The model under review builds one solid part; all positions refer to its coordinate system, in mm. Coordinates: 2 decimals unless noted, no trailing zeros. Use one line per item in the form item = value.
```python
from build123d import *

# Parameters (mm, degrees)
F0_W     = 282
F0_H     = 90
F0_R     = 1.85
F0_R_2   = 4
F1_DEPTH = 3


with BuildPart() as f1:
    # F0 (on Top) → F1 (new body)
    with BuildSketch(Plane.XY):
        Rectangle(F0_W, F0_H)
        with Locations((-136, -40)):
            Circle(F0_R, mode=Mode.SUBTRACT)
        with Locations((-120, -40)):
            Circle(F0_R, mode=Mode.SUBTRACT)
        with Locations((-104, -40)):
            Circle(F0_R, mode=Mode.SUBTRACT)
        with Locations((-88, -40)):
            Circle(F0_R, mode=Mode.SUBTRACT)
        with Locations((-72, -40)):
            Circle(F0_R, mode=Mode.SUBTRACT)
        with Locations((-56, -40)):
            Circle(F0_R, mode=Mode.SUBTRACT)
        with Locations((-40, -40)):
            Circle(F0_R, mode=Mode.SUBTRACT)
        with Locations((-24, -40)):
            Circle(F0_R, mode=Mode.SUBTRACT)
        with Locations((-8, -40)):
            Circle(F0_R, mode=Mode.SUBTRACT)
        with Locations((-128, -8)):
            Circle(F0_R, mode=Mode.SUBTRACT)
        with Locations((-96, -8)):
            Circle(F0_R, mode=Mode.SUBTRACT)
        with Locations((-64, -8)):
            Circle(F0_R, mode=Mode.SUBTRACT)
        with Locations((-32, -8)):
            Circle(F0_R, mode=Mode.SUBTRACT)
        with Locations((8, -40)):
            Circle(F0_R, mode=Mode.SUBTRACT)
        with Locations((24, -40)):
            Circle(F0_R, mode=Mode.SUBTRACT)
        with Locations((40, -40)):
            Circle(F0_R, mode=Mode.SUBTRACT)
        with Locations((56, -40)):
            Circle(F0_R, mode=Mode.SUBTRACT)
        with Locations((72, -40)):
            Circle(F0_R, mode=Mode.SUBTRACT)
        with Locations((88, -40)):
            Circle(F0_R, mode=Mode.SUBTRACT)
        with Locations((104, -40)):
            Circle(F0_R, mode=Mode.SUBTRACT)
        with Locations((120, -40)):
            Circle(F0_R, mode=Mode.SUBTRACT)
        with Locations((136, -40)):
            Circle(F0_R, mode=Mode.SUBTRACT)
        with Locations((0, -8)):
            Circle(F0_R, mode=Mode.SUBTRACT)
        with Locations((32, -8)):
            Circle(F0_R, mode=Mode.SUBTRACT)
        with Locations((64, -8)):
            Circle(F0_R, mode=Mode.SUBTRACT)
        with Locations((96, -8)):
            Circle(F0_R, mode=Mode.SUBTRACT)
        with Locations((128, -8)):
            Circle(F0_R, mode=Mode.SUBTRACT)
        with Locations((-136, 0)):
            Circle(F0_R, mode=Mode.SUBTRACT)
        with Locations((-128, 0)):
            Circle(F0_R_2, mode=Mode.SUBTRACT)
        with Locations((-120, 0)):
            Circle(F0_R, mode=Mode.SUBTRACT)
        with Locations((-128, 8)):
            Circle(F0_R, mode=Mode.SUBTRACT)
        with Locations((-104, 0)):
            Circle(F0_R, mode=Mode.SUBTRACT)
        with Locations((-96, 0)):
            Circle(F0_R_2, mode=Mode.SUBTRACT)
        with Locations((-88, 0)):
            Circle(F0_R, mode=Mode.SUBTRACT)
        with Locations((-72, 0)):
            Circle(F0_R, mode=Mode.SUBTRACT)
        with Locations((-96, 8)):
            Circle(F0_R, mode=Mode.SUBTRACT)
        with Locations((-64, 0)):
            Circle(F0_R_2, mode=Mode.SUBTRACT)
        with Locations((-56, 0)):
            Circle(F0_R, mode=Mode.SUBTRACT)
        with Locations((-40, 0)):
            Circle(F0_R, mode=Mode.SUBTRACT)
        with Locations((-64, 8)):
            Circle(F0_R, mode=Mode.SUBTRACT)
        with Locations((-32, 0)):
            Circle(F0_R_2, mode=Mode.SUBTRACT)
        with Locations((-24, 0)):
            Circle(F0_R, mode=Mode.SUBTRACT)
        with Locations((-8, 0)):
            Circle(F0_R, mode=Mode.SUBTRACT)
        with Locations((-32, 8)):
            Circle(F0_R, mode=Mode.SUBTRACT)
        with Locations((-136, 40)):
            Circle(F0_R, mode=Mode.SUBTRACT)
        with Locations((-120, 40)):
            Circle(F0_R, mode=Mode.SUBTRACT)
        with Locations((-104, 40)):
            Circle(F0_R, mode=Mode.SUBTRACT)
        with Locations((-88, 40)):
            Circle(F0_R, mode=Mode.SUBTRACT)
        with Locations((-72, 40)):
            Circle(F0_R, mode=Mode.SUBTRACT)
        with Locations((-56, 40)):
            Circle(F0_R, mode=Mode.SUBTRACT)
        with Locations((-40, 40)):
            Circle(F0_R, mode=Mode.SUBTRACT)
        with Locations((-24, 40)):
            Circle(F0_R, mode=Mode.SUBTRACT)
        with Locations((-8, 40)):
            Circle(F0_R, mode=Mode.SUBTRACT)
        Circle(F0_R_2, mode=Mode.SUBTRACT)
        with Locations((8, 0)):
            Circle(F0_R, mode=Mode.SUBTRACT)
        with Locations((24, 0)):
            Circle(F0_R, mode=Mode.SUBTRACT)
        with Locations((32, 0)):
            Circle(F0_R_2, mode=Mode.SUBTRACT)
        with Locations((0, 8)):
            Circle(F0_R, mode=Mode.SUBTRACT)
        with Locations((32, 8)):
            Circle(F0_R, mode=Mode.SUBTRACT)
        with Locations((40, 0)):
            Circle(F0_R, mode=Mode.SUBTRACT)
        with Locations((56, 0)):
            Circle(F0_R, mode=Mode.SUBTRACT)
        with Locations((64, 0)):
            Circle(F0_R_2, mode=Mode.SUBTRACT)
        with Locations((64, 8)):
            Circle(F0_R, mode=Mode.SUBTRACT)
        with Locations((72, 0)):
            Circle(F0_R, mode=Mode.SUBTRACT)
        with Locations((88, 0)):
            Circle(F0_R, mode=Mode.SUBTRACT)
        with Locations((96, 0)):
            Circle(F0_R_2, mode=Mode.SUBTRACT)
        with Locations((104, 0)):
            Circle(F0_R, mode=Mode.SUBTRACT)
        with Locations((96, 8)):
            Circle(F0_R, mode=Mode.SUBTRACT)
        with Locations((120, 0)):
            Circle(F0_R, mode=Mode.SUBTRACT)
        with Locations((128, 0)):
            Circle(F0_R_2, mode=Mode.SUBTRACT)
        with Locations((136, 0)):
            Circle(F0_R, mode=Mode.SUBTRACT)
        with Locations((128, 8)):
            Circle(F0_R, mode=Mode.SUBTRACT)
        with Locations((8, 40)):
            Circle(F0_R, mode=Mode.SUBTRACT)
        with Locations((24, 40)):
            Circle(F0_R, mode=Mode.SUBTRACT)
        with Locations((40, 40)):
            Circle(F0_R, mode=Mode.SUBTRACT)
        with Locations((56, 40)):
            Circle(F0_R, mode=Mode.SUBTRACT)
        with Locations((72, 40)):
            Circle(F0_R, mode=Mode.SUBTRACT)
        with Locations((88, 40)):
            Circle(F0_R, mode=Mode.SUBTRACT)
        with Locations((104, 40)):
            Circle(F0_R, mode=Mode.SUBTRACT)
        with Locations((120, 40)):
            Circle(F0_R, mode=Mode.SUBTRACT)
        with Locations((136, 40)):
            Circle(F0_R, mode=Mode.SUBTRACT)
    extrude(amount=F1_DEPTH)


solid = f1.part
```
1. Add section A-A (z = 0.85). Count the separate pieces of the cut face and the enclosed holes in it, then the cut area to 3 significant figures.
Response values:
separate_pieces = 1
enclosed_holes = 81
area = 24,200 mm^2
2. The part is to be moulded in two halves that separate along Y. For faces 1 (the face through (-2, 11, 0)), 2 (the face through (124, 0, 1)), say which applies: pulls with the +Y half, pulls with the -Y half, needs draft (parallel to the pull), parting line crosses it, or undercut.
Response values:
face_1 = needs draft
face_2 = undercut
3. Wall thickness on line 1 along Y through (x, z) = (120, 1.5); line 2 along Y through (x, z) = (64, 1.65); line 3 along Y through (x, z) = (61, 1.2): over which ranges is each line inside the solid? List them lowest first. Write a range as from..to.
Response values:
line_1 = -45..-41.85, -38.15..-1.85, 1.85..38.15, 41.85..45
line_2 = -45..-9.85, -6.15..-4, 4..6.15, 9.85..45
line_3 = -45..-2.65, 2.65..45
